from build123d import *

# Parameters (mm, degrees)
BOSS_EXTRUDE1_DEPTH = 3
SKETCH2_W           = 10
SKETCH2_H           = 2
CUT_EXTRUDE1_DEPTH  = 3
BOSS_EXTRUDE3_DEPTH = 3
SKETCH4_W           = 10
SKETCH4_H           = 2
CUT_EXTRUDE2_DEPTH  = 4
SKETCH5_R           = 8
CUT_EXTRUDE3_DEPTH  = 10


with BuildPart() as part:
    # Sketch1 → Boss-Extrude1 (new body)
    with BuildSketch(Plane(origin=(0, 0, 0), x_dir=(0, 0, -1), z_dir=(1, 0, 0))):
        Polygon((-3, 80.61), (-3, 106.39), (0, 106.39), (0, 113.14), (0, 116.39), (5, 116.39), (5, 116), (7, 116), (7, 116.39), (10, 116.39), (10, 120.61), (7, 120.61), (7, 121), (5, 121), (5, 120.61), (0, 120.61), (0, 124.11), (0, 130.61), (-3, 130.61), (-3, 156.39), (0, 156.39), (0, 159.89), (5, 159.89), (5, 159.5), (7, 159.5), (7, 159.89), (10, 159.89), (10, 164.11), (7, 164.11), (7, 164.5), (5, 164.5), (5, 164.11), (0, 164.11), (0, 167), (15.195, 167), (15.195, 162), (14.805, 162), (14.805, 160), (15.195, 160), (15.195, 157), (19.415, 157), (19.415, 160), (19.805, 160), (19.805, 162), (19.415, 162), (19.415, 167), (24.61, 167), (24.61, 170), (35.39, 170), (35.39, 167), (40.585, 167), (40.585, 162), (40.195, 162), (40.195, 160), (40.585, 160), (40.585, 157), (44.805, 157), (44.805, 160), (45.195, 160), (45.195, 162), (44.805, 162), (44.805, 167), (50, 167), (50, 0), (44.805, 0), (44.805, 5), (45.195, 5), (45.195, 7), (44.805, 7), (44.805, 10), (40.585, 10), (40.585, 7), (40.195, 7), (40.195, 5), (40.585, 5), (40.585, 0), (35.39, 0), (35.39, -3), (24.61, -3), (24.61, 0), (19.415, 0), (19.415, 5), (19.805, 5), (19.805, 7), (19.415, 7), (19.415, 10), (15.195, 10), (15.195, 7), (14.805, 7), (14.805, 5), (15.195, 5), (15.195, 0), (0, 0), (0, 8.24), (-3, 8.24), (-3, 15.87), (0, 15.87), (0, 23.5), (20, 23.5), (20, 63.5), (0, 63.5), (0, 66.39), (5, 66.39), (5, 66), (7, 66), (7, 66.39), (10, 66.39), (10, 70.61), (7, 70.61), (7, 71), (5, 71), (5, 70.61), (0, 70.61), (0, 80.61), align=None)
    extrude(amount=BOSS_EXTRUDE1_DEPTH)

    # Sketch2 → Cut-Extrude1 (cut)
    with BuildSketch(Plane(origin=(3, 0, 0), x_dir=(0, 0, -1), z_dir=(1, 0, 0))):
        with Locations((5, 1)):
            Rectangle(SKETCH2_W, SKETCH2_H)
    extrude(amount=-CUT_EXTRUDE1_DEPTH, mode=Mode.SUBTRACT)

    # Sketch3 → Boss-Extrude3 (add, through all)
    with BuildSketch(Plane(origin=(3, 0, 0), x_dir=(0, 0, -1), z_dir=(1, 0, 0))):
        Polygon((0, 164.11), (0, 159.89), (5, 159.89), (5, 159.5), (7, 159.5), (7, 159.89), (10, 159.89), (10, 164.11), (7, 164.11), (7, 164.5), (5, 164.5), (5, 164.11), align=None)
    extrude(amount=-BOSS_EXTRUDE3_DEPTH)

    # Sketch4 → Cut-Extrude2 (cut, through all)
    with BuildSketch(Plane(origin=(3, 0, 0), x_dir=(0, 0, -1), z_dir=(1, 0, 0))):
        with Locations((5, 166)):
            Rectangle(SKETCH4_W, SKETCH4_H)
    extrude(amount=-CUT_EXTRUDE2_DEPTH, mode=Mode.SUBTRACT)

    # Sketch5 → Cut-Extrude3 (cut)
    with BuildSketch(Plane(origin=(3, 0, 0), x_dir=(0, 0, -1), z_dir=(1, 0, 0))):
        with Locations((35, 30.5)):
            Circle(SKETCH5_R)
        with Locations((35, 56.5)):
            Circle(SKETCH5_R)
    extrude(amount=-CUT_EXTRUDE3_DEPTH, mode=Mode.SUBTRACT)


solid = part.part
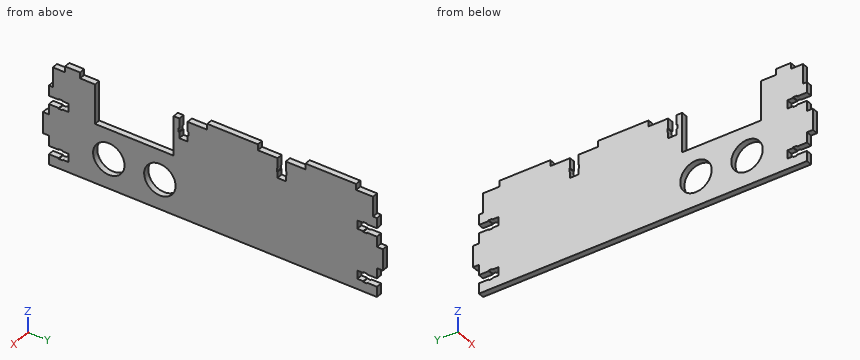
Input: part model. Units: mm. Frame: model coordinates. Coordinates: 2 decimals unless noted, no trailing zeros. Loops run counter-clockwise (first coordinate to the right, second up) from the corner with the lowest first, then second, coordinate; pieces in that order, holes last.
(1) Section D-D on y = 112. Return the cut outline in (x, z).
(2) Section B-B on z = -32.5. Return the cut outline in (x, y), then the cut area to 3 significant figures.
(3) Section C-C on x = 1.85. Count the separate pieces of the cut face and the enclosed holes in it, then the cut area to 3 significant figures.
(4) Material intervals for probe 1 along Y at (x, z) = (1.75, -35); probe 2 along Y at (x, z) = (0.6, 0.5); probe 3 along Y at (x, z) = (2.45, -5.5), sorted ascending.
(5) Section A-A on y = 30.5. Return the cut outline in (x, z).
(6) First-contact query: pin 1 Ø0.9 at (x, z) = (1.5, -3) entering from +Y; pin 2 Ø0.9 at (x, z) = (2, -48) entering from +Y; pin 3 Ø0.9 at (x, y) = (1.5, 4) entering from +Z. Flat tips, straight axial feed; report the tip coordinate or a pass-through.
Data:
1. outline: (0, -50) - (3, -50) - (3, 0) - (0, 0) - close
2. outline: (0, -3) - (3, -3) - (3, 22.9) - (0, 22.9) - close; (0, 38.1) - (3, 38.1) - (3, 48.9) - (0, 48.9) - close; (0, 64.1) - (3, 64.1) - (3, 170) - (0, 170) - close
2. area: 428 mm2
3. separate pieces: 1
3. enclosed holes: 2
3. area: 7,090 mm2
4. probe 1: y = -3 to 22.5, 38.5 to 48.5, 64.5 to 170
4. probe 2: y = 8.24 to 15.87, 80.61 to 106.39, 130.61 to 156.39
4. probe 3: y = 2 to 23.5, 63.5 to 66, 71 to 116, 121 to 165
5. outline: (0, -50) - (3, -50) - (3, -43) - (0, -43) - close; (0, -27) - (3, -27) - (3, -20) - (0, -20) - close
6. pin 1: stops at y = 165
6. pin 2: stops at y = 167
6. pin 3: stops at z = 0
